Solid Edge part; units mm, degrees
sketch "Sketch1" plane through (0, 0, 0) normal (0, 0, 1) x (1, 0, 0)
  circle A0 centre (0, 0) radius 6.1
extrude "Protrusion1" add sketch "Sketch1" along normal blind 10
sketch "Sketch2" plane through (0, 0, 10) normal (0, 0, 1) x (1, 0, 0)
  circle A0 centre (0, 0) radius 8
extrude "ExtrudedProtrusion_2" add sketch "Sketch2" along normal blind 6
sketch "Sketch3" plane through (0, 0, 16) normal (0, 0, 1) x (1, 0, 0)
  circle A0 centre (0, 0) radius 3
extrude "Cutout1" cut sketch "Sketch3" against normal through all
properties material "ABS Plastic, medium impact"
Verification items for the finished model (mm, model axes). A direction names the side the tool comes from. Give positions to 0.01 mm unless a question says otherwise; leave off trailing zeros. Write each loop counter-clockwise with the first axis right and the second up, starting at its lowest first coordinate (ties: lowest second). Pieces come first, ordered by that corner, then holes. Notation, with made-up numbers: (16.5, -15.75) - (75.5, -15.75) arc R13 cw to (75.5, 7.25) - close; hole circle Ø7 at (-1, 64). An arc over 180 degrees is marked (long way). Answer as CSV lines item,"result". Start each with the question number.
1. Sectioned sample at D-D (y = -4.25). Record the boundary of the cut face in (x, z).
2. Sectioned sample at A-A (y = 0). Record the boundary of the cut face in (x, z).
3. Draft check along X on faces 1 (the face through (1, 3, 0)), 2 (the face through (-3, 0, 8)), 3 (the face through (-6.094, -0.268, 4.93)). Enter one of: pulls with the +X half, pulls with the -X half, needs draft (parallel to the pull), parting line crosses it, or undercut.
4. Depth check by flat-ended pin: pin 1 (1.5 mm diameter, centred on y = 3.5, z = 1.5, fed in from +X); pin 2 (1 mm diameter, centred on y = -6, z = 4.5, fed in from +X); pin 3 (1 mm diameter, centred on x = 2, z = 11, fed in from -Y). Enter the tip coordinate at first touch or a pass-through.
5. Sectioned sample at B-B (x = 1.75). Record the boundary of the cut face in (y, z), then the cut area to 3 significant figures.
6. Sectioned sample at C-C (z = 8.5). Record the boundary of the cut face in (x, y).
7. Set-up check for faces 4 (the face through (-2, -6, 10)), 5 (the face through (-1.73, 7.81, 12.96)): record each of +Z, -Z, +X, -X, +Y, -Y from which the full face is reachable in a straight line by a thin tool's end or side.
8. Thickness scan on line 1 (Y direction, x = 0, z = 9.75); line 2 (Z direction, x = 6.25, y = 4); line 3 (X direction, y = 1.5, z = 7). Record the ranges inside material, lowest first.
Derived:
1,outline,"(-6.78, 10) - (-4.38, 10) - (-4.38, 0) - (4.38, 0) - (4.38, 10) - (6.78, 10) - (6.78, 16) - (-6.78, 16) - close"
2,outline,"(-8, 10) - (-6.1, 10) - (-6.1, 0) - (-3, 0) - (-3, 16) - (-8, 16) - close; (3, 0) - (6.1, 0) - (6.1, 10) - (8, 10) - (8, 16) - (3, 16) - close"
3,face 1,"needs draft"
3,face 2,"undercut"
3,face 3,"parting line crosses it"
4,pin 1,"x = 5.44"
4,pin 2,"x = 2.64"
4,pin 3,"y = -7.86"
5,outline,"(-7.81, 10) - (-5.84, 10) - (-5.84, 0) - (-2.44, 0) - (-2.44, 16) - (-7.81, 16) - close; (2.44, 0) - (5.84, 0) - (5.84, 10) - (7.81, 10) - (7.81, 16) - (2.44, 16) - close"
5,area,"133 mm²"
6,outline,"circle Ø12.2 at (0, 0); hole circle Ø6 at (0, 0)"
7,face 4,"-Z"
7,face 5,"+Z, -Z"
8,line 1,"-6.1 to -3, 3 to 6.1"
8,line 2,"10 to 16"
8,line 3,"-5.91 to -2.6, 2.6 to 5.91"
